from build123d import *

# Parameters (mm, degrees)
F1_DEPTH = 63.5
F0_W     = 25.4
F0_H     = 4.7752
F0_H_2   = 19.05
F0_H_3   = 4.7498
F2_DEPTH = 25.4


with BuildPart() as f1:
    # F0 (on Front) → F1 (new body, symmetric)
    with BuildSketch(Plane.XZ):
        Polygon((-41.275, -9.525), (41.275, -9.525), (41.275, 9.525), (22.225, 9.525), (-41.275, 9.525), align=None)
    extrude(amount=F1_DEPTH, both=True)

    # F0 (on Front) → F2 (join, symmetric)
    with BuildSketch(Plane.XZ):
        Polygon((-41.275, -9.525), (41.275, -9.525), (41.275, 9.525), (22.225, 9.525), (-41.275, 9.525), align=None)
        with BuildLine():
            Line((22.225, 9.525), (41.275, 9.525))
            Line((41.275, 9.525), (41.275, 27.0002))
            ThreePointArc((41.275, 27.0002), (45.9246798487, 38.2255201513), (57.15, 42.8752))
            Line((57.15, 42.8752), (60.325, 42.8752))
            Line((60.325, 42.8752), (60.325, 61.9252))
            Line((60.325, 61.9252), (57.15, 61.9252))
            add(Edge.make_bspline(
                [(54.7155660835, 61.8402510405), (55.5417802596, 61.8812323072), (56.3536366675, 61.9096388708), (57.15, 61.9252)],
                knots=[108.932762341, 108.932762341, 108.932762341, 108.932762341, 111.5045361635, 111.5045361635, 111.5045361635, 111.5045361635], degree=3))
            ThreePointArc((54.7155660835, 61.8402510405), (31.6080910117, 50.8196565478), (22.225, 27.0002))
            Line((22.225, 27.0002), (22.225, 9.525))
        make_face()
        with BuildLine():
            add(Edge.make_bspline(
                [(-41.275, 9.525), (-41.0359900889, 35.8080333055), (19.7195677178, 60.1044053224), (54.7155660835, 61.8402510405)],
                knots=[0, 0, 0, 0, 108.932762341, 108.932762341, 108.932762341, 108.932762341], degree=3))
            Line((-41.275, 9.525), (22.225, 9.525))
            Line((22.225, 9.525), (22.225, 27.0002))
            ThreePointArc((22.225, 27.0002), (31.6080910117, 50.8196565478), (54.7155660835, 61.8402510405))
        make_face()
        with BuildLine():
            ThreePointArc((57.15, 61.9252), (55.9320421991, 61.9039562992), (54.7155660835, 61.8402510405))
            add(Edge.make_bspline(
                [(54.7155660835, 61.8402510405), (55.5417802596, 61.8812323072), (56.3536366675, 61.9096388708), (57.15, 61.9252)],
                knots=[108.932762341, 108.932762341, 108.932762341, 108.932762341, 111.5045361635, 111.5045361635, 111.5045361635, 111.5045361635], degree=3))
        make_face()
        with Locations((73.025, 40.4876)):
            Rectangle(F0_W, F0_H)
        with Locations((73.025, 52.4002)):
            Rectangle(F0_W, F0_H_2)
        with Locations((73.025, 64.3001)):
            Rectangle(F0_W, F0_H_3)
        Polygon((85.725, 61.9252), (85.725, 42.8752), (85.725, 38.1), (111.125, 38.1), (111.125, 66.675), (85.725, 66.675), align=None)
    extrude(amount=F2_DEPTH, both=True)


solid = f1.part
Here's how the part is built. I have some questions about the finished solid (model axes, mm). A direction names the side the tool comes from. Round coordinates to 2 decimals unless told otherwise and drop trailing zeros. Write each loop counter-clockwise with the first axis right and the second up, starting at its lowest first coordinate (ties: lowest second). Pieces come first, ordered by that corner, then holes. Notation, with made-up numbers: (-38, 62.25) -> (2, 62.25) arc R21 ccw to (2, 101.25) -> close; hole circle Ø9 at (0, 26). An arc over 180 degrees is marked (long way). One line per item, written item: value.
1) I'm going to push flat-ended pins straight in: pin 1 Ø17 at (x, z) = (50.5, 41.5) entering from -Y; pin 2 Ø12 at (x, z) = (-14.5, 53) entering from +Y; pin 3 Ø11 at (y, z) = (-30.5, 17) entering from +X (3 decimals); pin 4 Ø3 at (y, z) = (21, 37) entering from -X. Where does each tip first touch, or does it pass through?
Filled sheet:
pin 1: stops at y = -25.4
pin 2: passes through
pin 3: stops at x = 41.275
pin 4: stops at x = -22.5
2) Suppose I cut it at B-B on x = 62.5. List the corners of the cut face in (y, z) for me (3 decimals).
Filled sheet:
outline: (-25.4, 38.1) -> (25.4, 38.1) -> (25.4, 66.675) -> (-25.4, 66.675) -> close
3) If I drill on line 1 (Y direction, x = 8, z = 38); line 2 (X direction, y = -33, z = 4) (3 decimals); line 3 (Z direction, x = 82.5, y = -10) (3 decimals), over which ranges is the centre line in solid material (lowest first)? Write a range as [from, to].
Filled sheet:
line 1: y = [-25.4, 25.4]
line 2: x = [-41.275, 41.275]
line 3: z = [38.1, 66.675]
4) Suppose I cut it at A-A on y = -45. List the corners of the cut face in (x, z) for me (3 decimals), plus the area to 3 significant figures.
Filled sheet:
outline: (-41.275, -9.525) -> (41.275, -9.525) -> (41.275, 9.525) -> (-41.275, 9.525) -> close
area: 1,570 mm2
5) We'd pull the mould along X, two halves only. Please class faces 6 (the face through (-41.275, -1, 0)), 7 (the face through (1, 44, 9.525)), 8 (the face through (45.8, -0.4, 38.1)): released by +X, released by -X, zero draft, split by the parting line, or undercut.
Filled sheet:
face 6: released by -X
face 7: zero draft
face 8: undercut
6) For faces 1 (the face through (41.275, -1, 4)), 2 (the face through (34, 25.4, 39)), 3 (the face through (60.325, 0, 64)), 4 (the face through (60.325, 0, 40)), 5 (the face through (1, -45, 9.525)), which set-ups out of +Z, -Z, +X, -X, +Y, -Y let a thin tool reach every point of the face, with its end or its side?
Filled sheet:
face 1: -Z, +X, +Y, -Y
face 2: +Z, +X, -X, +Y
face 3: +Z, -X, +Y, -Y
face 4: -Z, +Y, -Y
face 5: +Z, +X, -X, -Y
